from build123d import *

# Parameters (mm, degrees)
CROQUIS1_4_W              = 50.8
CROQUIS1_4_H              = 50.8
SALIENTE_EXTRUIR3_DEPTH   = 240
SALIENTE_EXTRUIR3_2_DEPTH = 240
SALIENTE_EXTRUIR3_3_DEPTH = 240
SALIENTE_EXTRUIR3_4_DEPTH = 240
SALIENTE_EXTRUIR4_START   = -240
CROQUIS1_5_W              = 346.8
CROQUIS1_5_H              = 596.8
CROQUIS1_5_W_2            = 50.8
CROQUIS1_5_H_2            = 50.8
SALIENTE_EXTRUIR4_DEPTH   = 40


with BuildPart() as part:
    # Croquis1<4> → Saliente-Extruir3 (new body)
    with BuildSketch(Plane(origin=(0, 0, 0), x_dir=(1, 0, 0), z_dir=(0, 1, 0))):
        with Locations((-423, -323.8)):
            Rectangle(CROQUIS1_4_W, CROQUIS1_4_H)
    extrude(amount=-SALIENTE_EXTRUIR3_DEPTH)



with BuildPart() as body_2:
    # Croquis1<4> → Saliente-Extruir3 2 (new body)
    with BuildSketch(Plane(origin=(0, 0, 0), x_dir=(1, 0, 0), z_dir=(0, 1, 0))):
        with Locations((-423, 323.8)):
            Rectangle(CROQUIS1_4_W, CROQUIS1_4_H)
    extrude(amount=-SALIENTE_EXTRUIR3_2_DEPTH)


with BuildPart() as body_3:
    # Croquis1<4> → Saliente-Extruir3 3 (new body)
    with BuildSketch(Plane(origin=(0, 0, 0), x_dir=(1, 0, 0), z_dir=(0, 1, 0))):
        with Locations((-25.4, 323.8)):
            Rectangle(CROQUIS1_4_W, CROQUIS1_4_H)
    extrude(amount=-SALIENTE_EXTRUIR3_3_DEPTH)


with BuildPart() as body_4:
    # Croquis1<4> → Saliente-Extruir3 4 (new body)
    with BuildSketch(Plane(origin=(0, 0, 0), x_dir=(1, 0, 0), z_dir=(0, 1, 0))):
        with Locations((-25.4, -323.8)):
            Rectangle(CROQUIS1_4_W, CROQUIS1_4_H)
    extrude(amount=-SALIENTE_EXTRUIR3_4_DEPTH)


with BuildPart() as part_1:
    add(part.part)

    add(body_2.part)  # Saliente-Extruir4 merges body 2

    add(body_3.part)  # Saliente-Extruir4 merges body 3

    add(body_4.part)  # Saliente-Extruir4 merges body 4
    # Croquis1<5> → Saliente-Extruir4 (add)
    with BuildSketch(Plane(origin=(0, 0, 0), x_dir=(1, 0, 0), z_dir=(0, 1, 0)).offset(SALIENTE_EXTRUIR4_START)):
        with Locations((-224.2, 0)):
            Rectangle(CROQUIS1_5_W, CROQUIS1_5_H)
        with Locations((-25.4, 0)):
            Rectangle(CROQUIS1_5_W_2, CROQUIS1_5_H)
        with Locations((-224.2, -323.8)):
            Rectangle(CROQUIS1_5_W, CROQUIS1_5_H_2)
        with Locations((-423, 0)):
            Rectangle(CROQUIS1_5_W_2, CROQUIS1_5_H)
        with Locations((-224.2, 323.8)):
            Rectangle(CROQUIS1_5_W, CROQUIS1_5_H_2)
        with Locations((-423, 323.8)):
            Rectangle(CROQUIS1_5_W_2, CROQUIS1_5_H_2)
        with Locations((-25.4, 323.8)):
            Rectangle(CROQUIS1_5_W_2, CROQUIS1_5_H_2)
        with Locations((-25.4, -323.8)):
            Rectangle(CROQUIS1_5_W_2, CROQUIS1_5_H_2)
        with Locations((-423, -323.8)):
            Rectangle(CROQUIS1_5_W_2, CROQUIS1_5_H_2)
    extrude(amount=SALIENTE_EXTRUIR4_DEPTH)


solid = part_1.part
Design review of the part built by this model. Coordinates are the model's own, in mm. A direction names the side the tool comes from. Round coordinates to 2 decimals unless told otherwise and drop trailing zeros. Loops run counter-clockwise (first coordinate to the right, second up) from the corner with the lowest first, then second, coordinate; pieces in that order, holes last. Notation, with made-up numbers: (18.25, -32.5) -> (45.25, -32.5) arc R26 ccw to (45.25, 5.5) -> close; hole circle Ø7 at (60, 47.5). An arc over 180 degrees is marked (long way). Use one line per item in the form item = value. Start each with the question number.
Q1. We need section B-B on z = -151.5. Give the boundary of the cut face in (x, y).
Q2. We need section A-A on y = -119. Give the boundary of the cut face in (x, z).
Q3. Draft analysis for pull direction Z (two halves, no side actions). For faces 1 (the face through (-26, -99, 298.4)), 2 (the face through (-221, -202, -349.2)), 3 (the face through (-423, 0, 323)), state which applies: +Z half, -Z half, draft (parallel to the pull), parting line (faces both ways), or undercut.
Q4. We need section C-C on x = -211.5. Give the boundary of the cut face in (y, z).
Q5. For pin 1 Ø6 at (x, z) = (-311, 208) entering from +Y, flat-tipped, find the tip position at first contact; note if it passes through.
Q6. Machinability: for faces 4 (the face through (-50.8, -99, 324)), 5 (the face through (0, -208, -24)), 6 (the face through (-26, -99, -298.4)), which of the approach directions +Z, -Z, +X, -X, +Y, -Y give a long, thin tool a straight path to every point of the face, cutting with its end or side? Answer none if there is none.
Q7. Wall thickness on line 1 along Z through (x, y) = (-34, -196); line 2 along Y through (x, z) = (-304.5, 159): over which ranges is each line inside the solid? List them lowest first. Write a range as [from, to].
Calculated:
q1.outline = (-448.4, -240) -> (0, -240) -> (0, -200) -> (-448.4, -200) -> close
q2.outline = (-448.4, -349.2) -> (-397.6, -349.2) -> (-397.6, -298.4) -> (-448.4, -298.4) -> close; (-448.4, 298.4) -> (-397.6, 298.4) -> (-397.6, 349.2) -> (-448.4, 349.2) -> close; (-50.8, -349.2) -> (0, -349.2) -> (0, -298.4) -> (-50.8, -298.4) -> close; (-50.8, 298.4) -> (0, 298.4) -> (0, 349.2) -> (-50.8, 349.2) -> close
q3.face_1 = undercut
q3.face_2 = -Z half
q3.face_3 = draft
q4.outline = (-240, -349.2) -> (-200, -349.2) -> (-200, 349.2) -> (-240, 349.2) -> close
q5.pin_1 = -200
q6.face_4 = +Z, -Z, +Y
q6.face_5 = +Z, -Z, +X, +Y, -Y
q6.face_6 = +X, -X, +Y
q7.line_1 = [-349.2, -298.4], [298.4, 349.2]
q7.line_2 = [-240, -200]
